from build123d import *

# Parameters (mm, degrees)
SKETCH_1_W          = 40
SKETCH_1_H          = 40
SKETCH_1_R          = 15
EXTRUDE_1_DEPTH     = 40
SKETCH_2_R          = 1.5
CUT_EXTRUDE_1_DEPTH = 61
SKETCH_3_R          = 4
EXTRUDE_2_DEPTH     = 8
FILLET_1_R          = 11


with BuildPart() as part:
    # 草圖1 → 填料-伸長1 (new body)
    with BuildSketch(Plane(origin=(0, 0, 0), x_dir=(1, 0, 0), z_dir=(0, 1, 0))):
        Rectangle(SKETCH_1_W, SKETCH_1_H)
        with Locations(Location((0, 0, 0), (0, 0, 270))):
            Circle(SKETCH_1_R, mode=Mode.SUBTRACT)
    extrude(amount=EXTRUDE_1_DEPTH)

    # 草圖2 → 除料-伸長1 (cut, through all)
    with BuildSketch(Plane.XY.offset(20)):
        with Locations((0, 10)):
            Circle(SKETCH_2_R)
        with Locations((0, 30)):
            Circle(SKETCH_2_R)
    extrude(amount=-CUT_EXTRUDE_1_DEPTH, mode=Mode.SUBTRACT)

    # 草圖3 → 填料-伸長2 (add)
    with BuildSketch(Plane(origin=(20, 0, 0), x_dir=(0, 0, -1), z_dir=(1, 0, 0))):
        with BuildLine():
            Line((-20, 0), (-31, 0))
            ThreePointArc((-31, 0), (-38, 7), (-31, 14))
            Line((-31, 14), (-20, 14))
            Line((-20, 14), (-20, 0))
        make_face()
        with Locations((-31, 7)):
            Circle(SKETCH_3_R, mode=Mode.SUBTRACT)
    extrude(amount=-EXTRUDE_2_DEPTH)

    # 圓角1
    fillet_1_edges = [part.edges().sort_by_distance(p)[0] for p in [
        (16, 14, 20),
    ]]
    fillet(fillet_1_edges, radius=FILLET_1_R - 0.0001)  # a hair under: the kernel refuses the full size


solid = part.part
Source: CAD feature listing. Evaluate the final solid. Frame: model axes, mm. A direction names the side the tool comes from. Give positions to 0.01 mm unless a question says otherwise; leave off trailing zeros. Write each loop counter-clockwise with the first axis right and the second up, starting at its lowest first coordinate (ties: lowest second). Pieces come first, ordered by that corner, then holes. Notation, with made-up numbers: M 14.5,-40 L 65.5,-40 A25 cw 65.5,-15 Z; hole C -3,-30 d4. An arc over 180 degrees is marked long. Return JSON: item names as keys, results as strings. Group by question number.
1) Set-up query: faces 1 (the face through (0, 20, -20)), 2 (the face through (12, 10, 27)). Return all of +Z, -Z, +X, -X, +Y, -Y with unobstructed straight access to the full face (end or side cutting, diameter ignored); none if empty.
2) Draft query along X for faces 3 (the face through (-0.325, 8.536, -17.426)), 4 (the face through (20, 20, 2)), 5 (the face through (0, 0, 16)). Return one class per face: released by +X, released by -X, zero draft, split by the parting line, or undercut.
3) Ray query, L1, parallel to Z at x = 0, y = 13; L2, parallel to Y at x = 15.25, z = 31; L3, parallel to X at y = 10, z = 17. Return the intervals inside material, ascending.
4) Cut plane A-A, the plane z = 0. Output: boundary loops of the cut face in (x, y), then the cut area to 3 significant figures.
5) Cut plane D-D, the plane x = 0. Output: boundary loops of the cut face in (y, z).
6) Cut plane B-B, the plane x = -9. Output: boundary loops of the cut face in (y, z).
7) Cut plane C-C, the plane y = 26. Output: boundary loops of the cut face in (x, z), then the cut area to 3 significant figures.
8) First-contact query: pin 1 Ø8 at (x, y) = (-11, 27.5) entering from +Z; pin 2 Ø14.5 at (y, z) = (16.5, 28.5) entering from -X. Flat tips, straight axial feed; report the tip coordinate or a pass-through.
Data:
{
 "1": {"face 1": "-Z, +X, -X, +Y, -Y", "face 2": "+Z, -X, +Y, -Y"},
 "2": {"face 3": "undercut", "face 4": "released by +X", "face 5": "zero draft"},
 "3": {"L1": "z = -20 to -15, 15 to 20", "L2": "y = 0 to 3, 11 to 14", "L3": "x = -20 to -1.5, 1.5 to 20"},
 "4": {"outline": "M -20,0 L -15,0 L -15,40 L -20,40 Z; M 15,0 L 20,0 L 20,40 L 15,40 Z", "area": "400 mm²"},
 "5": {"outline": "M 0,-20 L 8.5,-20 L 8.5,-15 L 0,-15 Z; M 0,15 L 8.5,15 L 8.5,20 L 0,20 Z; M 11.5,-20 L 28.5,-20 L 28.5,-15 L 11.5,-15 Z; M 11.5,15 L 28.5,15 L 28.5,20 L 11.5,20 Z; M 31.5,-20 L 40,-20 L 40,-15 L 31.5,-15 Z; M 31.5,15 L 40,15 L 40,20 L 31.5,20 Z"},
 "6": {"outline": "M 0,-20 L 40,-20 L 40,-12 L 0,-12 Z; M 0,12 L 40,12 L 40,20 L 0,20 Z"},
 "7": {"outline": "M -20,-20 L 20,-20 L 20,20 L -20,20 Z; hole C 0,0 d30", "area": "893 mm²"},
 "8": {"pin 1": "stops at z = 20", "pin 2": "stops at x = 12"}
}
